from build123d import *

# Parameters (mm, degrees)
SKETCH1_R           = 24.765
BOSS_EXTRUDE1_DEPTH = 121.031
SKETCH3_R           = 24.765
BOSS_EXTRUDE2_DEPTH = 38.1
CHAMFER1_SIZE       = 19.05


with BuildPart() as part:
    # Sketch1 → Boss-Extrude1 (new body)
    with BuildSketch(Plane(origin=(0, 0, 0), x_dir=(0, 0, -1), z_dir=(1, 0, 0))):
        Circle(SKETCH1_R)
    extrude(amount=BOSS_EXTRUDE1_DEPTH)

    # Sketch3 → Boss-Extrude2 (add)
    with BuildSketch(Plane.ZY):
        Circle(SKETCH3_R)
    extrude(amount=BOSS_EXTRUDE2_DEPTH)

    # Chamfer1
    chamfer1_edges = [part.edges().sort_by_distance(p)[0] for p in [
        (-38.1, 0, -24.765),
    ]]
    chamfer(chamfer1_edges, length=CHAMFER1_SIZE)


solid = part.part
Here's how the part is built. I have some questions about the finished solid (model axes, mm). Give positions to 0.01 mm unless a question says otherwise; leave off trailing zeros. Order: outer loops, then holes, each group sorted by start corner. A loop starts at its lowest first (then second) coordinate and runs counter-clockwise, first axis right, second up. Notation, with made-up numbers: M 49,17.5 L 63,17.5 A22 ccw 63,40.5 Z; hole C -3,5 d6. An arc over 180 degrees is marked long. Answer as a JSON object with one key per item and string values. Group by question number.
1) I'm going to push flat-ended pins straight in: pin 1 Ø2 at (x, y) = (91, 2) entering from -Z; pin 2 Ø4 at (x, y) = (12.5, 6) entering from -Z; pin 3 Ø10 at (x, y) = (38, 7) entering from +Z; pin 4 Ø12 at (x, y) = (87.5, -4) entering from +Z (3 decimals). Where does each tip first touch, or does it pass through?
2) Suppose I cut it at C-C, the plane x = 87. Write out the boundary of the cut face in (y, z) (3 decimals), plus the area to 3 significant figures.
3) Suppose I cut it at A-A, the plane y = 0. Write out the boundary of the cut face in (x, z) (3 decimals).
4) Please list where these lines run through material, in increasing order: L1, parallel to Z at x = 3, y = -1.5; L2, parallel to Y at x = 50, z = 3; L3, parallel to Z at x = 36.5, y = 6.5. Write a range as [from, to].
Results found:
{
 "1": {"pin 1": "z = -24.74", "pin 2": "z = -24.44", "pin 3": "z = 24.68", "pin 4": "z = 24.765"},
 "2": {"outline": "C 0,0 d49.53", "area": "1,930 mm²"},
 "3": {"outline": "M -38.1,-5.715 L -19.05,-24.765 L 121.031,-24.765 L 121.031,24.765 L -19.05,24.765 L -38.1,5.715 Z"},
 "4": {"L1": "[-24.72, 24.72]", "L2": "[-24.58, 24.58]", "L3": "[-23.9, 23.9]"}
}
